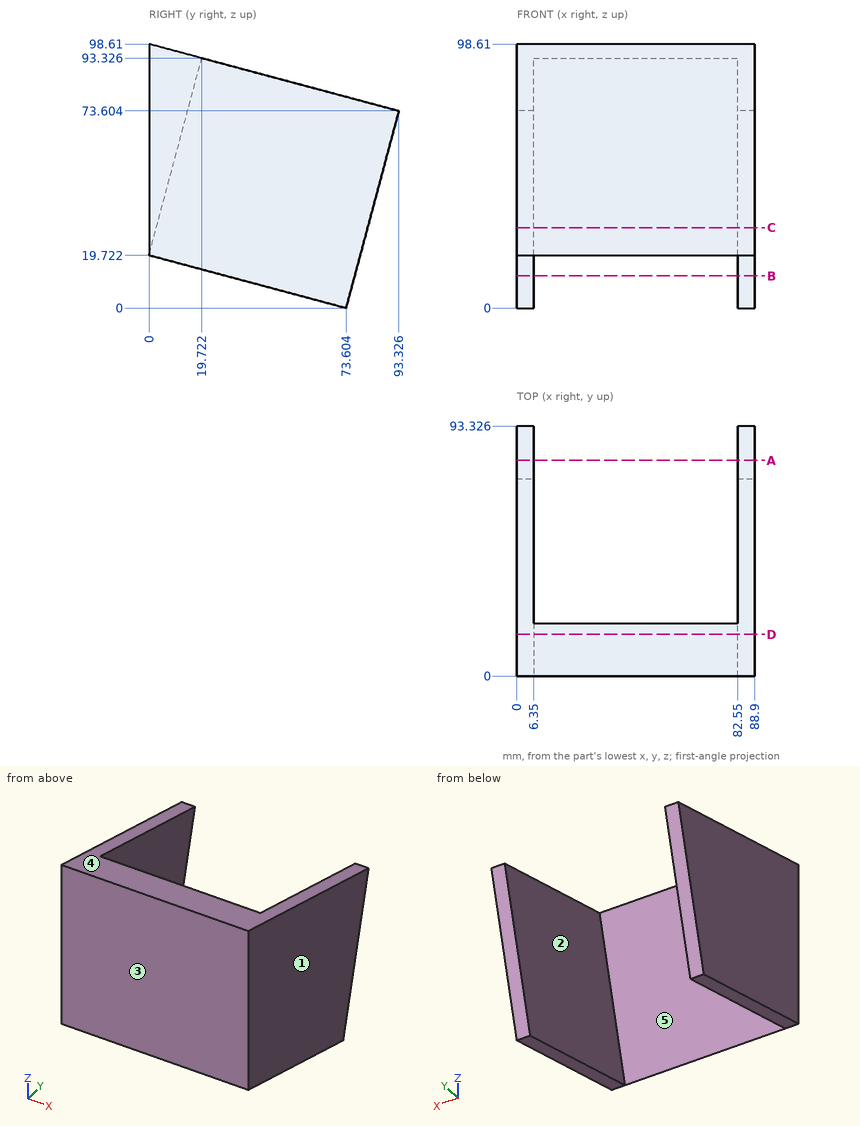
For this review, use the dimensioned drawing (mm, ordinates from the lowest corner) and the shaded views. A direction names the side the tool comes from. Round coordinates to 2 decimals unless told otherwise and drop trailing zeros. Write each loop counter-clockwise with the first axis right and the second up, starting at its lowest first coordinate (ties: lowest second). Pieces come first, ordered by that corner, then holes. Notation, with made-up numbers: (62.25, -40) - (117.25, -40) arc R25 cw to (117.25, -7) - close; hole circle Ø2 at (30, -20). An arc over 180 degrees is marked (long way). Answer as a JSON object with one key per item and string values.
1. To check wall thickness, follow line 1 along X through (y, z) = (65.5, 37); line 2 along Y through (x, z) = (18.5, 77); line 3 along Y through (x, z) = (69, 72). State the ranges of each line that lie inside material, in increasing order.
Response values:
{"line 1": "x = 0 to 6.35, 82.55 to 88.9", "line 2": "y = 0 to 15.35", "line 3": "y = 0 to 14.01"}
2. We need section C-C on z = 30. Give the boundary of the cut face in (x, y).
Response values:
{"outline": "(0, 0) - (88.9, 0) - (88.9, 81.64) - (82.55, 81.64) - (82.55, 2.75) - (6.35, 2.75) - (6.35, 81.64) - (0, 81.64) - close"}
3. For pin 1 Ø6 at (y, z) = (9.5, 30.5) entering from -X; pin 2 Ø2 at (x, z) = (21.5, 83.5) entering from +Y; pin 3 Ø2 at (x, z) = (58.5, 43.5) entering from +Y; pin 4 Ø12 at (x, z) = (19, 49.5) entering from +Y, all flat-tipped, find the tip position at first contact; note any pin that passes through.
Response values:
{"pin 1": "stops at x = 0", "pin 2": "stops at y = 17.36", "pin 3": "stops at y = 6.64", "pin 4": "stops at y = 9.59"}
4. Draft analysis for pull direction X (two halves, no side actions). For the marked faces 1, 2 and 3, state which applies: +X half, -X half, draft (parallel to the pull), parting line (faces both ways), or undercut.
Response values:
{"face 1": "+X half", "face 2": "undercut", "face 3": "draft"}
5. We need section B-B on z = 12. Give the boundary of the cut face in (x, y).
Response values:
{"outline": "(0, 28.82) - (6.35, 28.82) - (6.35, 76.82) - (0, 76.82) - close; (82.55, 28.82) - (88.9, 28.82) - (88.9, 76.82) - (82.55, 76.82) - close"}
6. We need section D-D on y = 15.5. Give the boundary of the cut face in (x, z), then the cut area to 3 significant figures.
Response values:
{"outline": "(0, 15.57) - (6.35, 15.57) - (6.35, 77.57) - (82.55, 77.57) - (82.55, 15.57) - (88.9, 15.57) - (88.9, 94.46) - (0, 94.46) - close", "area": "2,290 mm2"}
7. We need section A-A on y = 80.5. Give the boundary of the cut face in (x, z).
Response values:
{"outline": "(0, 25.74) - (6.35, 25.74) - (6.35, 77.04) - (0, 77.04) - close; (82.55, 25.74) - (88.9, 25.74) - (88.9, 77.04) - (82.55, 77.04) - close"}
8. Tool access review of the marked faces 4 and 5: name each direction out of +Z, -Z, +X, -X, +Y, -Y from which nothing blocks a thin tool from reaching the whole face with its end or side.
Response values:
{"face 4": "+Z, +X, -X, +Y", "face 5": "-Z, +Y"}
